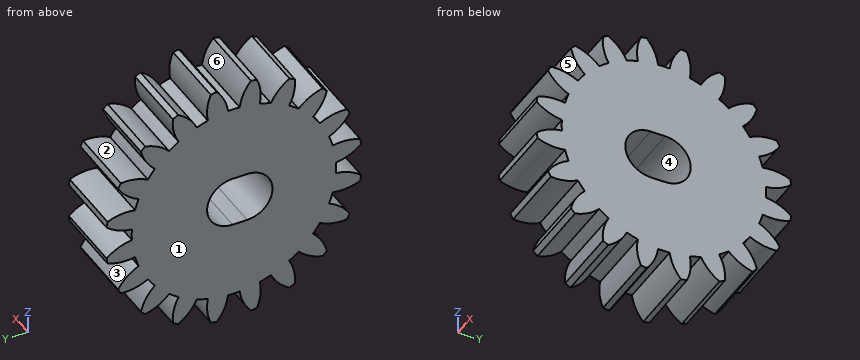
from build123d import *

# Parameters (mm, degrees)
EXTRUDE_1_DEPTH = 6


with BuildPart() as part:
    # Эскиз1 → Бобышка-Вытянуть1 (new body)
    with BuildSketch(Plane(origin=(0.204923016, 3.152126199, 1.20502958), x_dir=(0, 0, -1), z_dir=(1, 0, 0))):
        with BuildLine():
            ThreePointArc((-9.696984117, -1.687169764), (-8.686522764, -2.334065374), (-7.529675738, -2.652202191))
            ThreePointArc((-7.529675738, -2.652202191), (-7.54397042, -3.152126199), (-7.529675738, -3.652050206))
            ThreePointArc((-7.529675738, -3.652050206), (-8.686522764, -3.970187024), (-9.696984117, -4.617082634))
            ThreePointArc((-9.696984117, -4.617082634), (-9.659542166, -4.872905314), (-9.616098021, -5.12777734))
            ThreePointArc((-9.616098021, -5.12777734), (-8.45519043, -5.430761896), (-7.256653844, -5.375842598))
            ThreePointArc((-7.256653844, -5.375842598), (-7.115763881, -5.855715883), (-6.947683816, -6.326754568))
            ThreePointArc((-6.947683816, -6.326754568), (-7.949601035, -6.986806052), (-8.710705152, -7.914290068))
            ThreePointArc((-8.710705152, -7.914290068), (-8.596042186, -8.146021696), (-8.475964561, -8.374994418))
            ThreePointArc((-8.475964561, -8.374994418), (-7.278248455, -8.304409679), (-6.155343422, -7.88181015))
            ThreePointArc((-6.155343422, -7.88181015), (-5.873060104, -8.294659371), (-5.567647504, -8.690704186))
            ThreePointArc((-5.567647504, -8.690704186), (-6.316560278, -9.628059899), (-6.753804986, -10.745343722))
            ThreePointArc((-6.753804986, -10.745343722), (-6.573145013, -10.930300792), (-6.388187943, -11.110960765))
            ThreePointArc((-6.388187943, -11.110960765), (-5.27090412, -10.673716057), (-4.333548407, -9.924803283))
            ThreePointArc((-4.333548407, -9.924803283), (-3.937503592, -10.230215883), (-3.524654371, -10.512499201))
            ThreePointArc((-3.524654371, -10.512499201), (-3.9472539, -11.635404234), (-4.017838639, -12.83312034))
            ThreePointArc((-4.017838639, -12.83312034), (-3.788865917, -12.953197965), (-3.557134289, -13.067860931))
            ThreePointArc((-3.557134289, -13.067860931), (-2.629650273, -12.306756814), (-1.969598789, -11.304839595))
            ThreePointArc((-1.969598789, -11.304839595), (-1.498560104, -11.47291966), (-1.018686819, -11.613809623))
            ThreePointArc((-1.018686819, -11.613809623), (-1.073606117, -12.812346209), (-0.770621561, -13.9732538))
            ThreePointArc((-0.770621561, -13.9732538), (-0.515749535, -14.016697945), (-0.259926855, -14.054139896))
            ThreePointArc((-0.259926855, -14.054139896), (0.386968755, -13.043678543), (0.705105573, -11.886831517))
            ThreePointArc((0.705105573, -11.886831517), (1.20502958, -11.901126199), (1.704953588, -11.886831517))
            ThreePointArc((1.704953588, -11.886831517), (2.023090405, -13.043678543), (2.669986015, -14.054139896))
            ThreePointArc((2.669986015, -14.054139896), (2.925808695, -14.016697945), (3.180680722, -13.9732538))
            ThreePointArc((3.180680722, -13.9732538), (3.483665277, -12.812346209), (3.428745979, -11.613809623))
            ThreePointArc((3.428745979, -11.613809623), (3.908619264, -11.47291966), (4.379657949, -11.304839595))
            ThreePointArc((4.379657949, -11.304839595), (5.039709433, -12.306756814), (5.967193449, -13.067860931))
            ThreePointArc((5.967193449, -13.067860931), (6.198925077, -12.953197965), (6.427897799, -12.83312034))
            ThreePointArc((6.427897799, -12.83312034), (6.35731306, -11.635404234), (5.934713531, -10.512499201))
            ThreePointArc((5.934713531, -10.512499201), (6.347562752, -10.230215883), (6.743607567, -9.924803283))
            ThreePointArc((6.743607567, -9.924803283), (7.68096328, -10.673716057), (8.798247103, -11.110960765))
            ThreePointArc((8.798247103, -11.110960765), (8.983204173, -10.930300792), (9.163864146, -10.745343722))
            ThreePointArc((9.163864146, -10.745343722), (8.726619438, -9.628059899), (7.977706664, -8.690704186))
            ThreePointArc((7.977706664, -8.690704186), (8.283119264, -8.294659371), (8.565402582, -7.88181015))
            ThreePointArc((8.565402582, -7.88181015), (9.688307615, -8.304409679), (10.886023721, -8.374994418))
            ThreePointArc((10.886023721, -8.374994418), (11.006101346, -8.146021696), (11.120764313, -7.914290068))
            ThreePointArc((11.120764313, -7.914290068), (10.359660195, -6.986806052), (9.357742976, -6.326754568))
            ThreePointArc((9.357742976, -6.326754568), (9.525823041, -5.855715883), (9.666713005, -5.375842598))
            ThreePointArc((9.666713005, -5.375842598), (10.86524959, -5.430761896), (12.026157182, -5.12777734))
            ThreePointArc((12.026157182, -5.12777734), (12.069601327, -4.872905314), (12.107043277, -4.617082634))
            ThreePointArc((12.107043277, -4.617082634), (11.096581924, -3.970187024), (9.939734898, -3.652050206))
            ThreePointArc((9.939734898, -3.652050206), (9.95402958, -3.152126199), (9.939734898, -2.652202191))
            ThreePointArc((9.939734898, -2.652202191), (11.096581924, -2.334065374), (12.107043277, -1.687169764))
            ThreePointArc((12.107043277, -1.687169764), (12.069601327, -1.431347083), (12.026157182, -1.176475057))
            ThreePointArc((12.026157182, -1.176475057), (10.86524959, -0.873490502), (9.666713005, -0.9284098))
            ThreePointArc((9.666713005, -0.9284098), (9.525823041, -0.448536515), (9.357742976, 0.02250217))
            ThreePointArc((9.357742976, 0.02250217), (10.359660195, 0.682553654), (11.120764313, 1.61003767))
            ThreePointArc((11.120764313, 1.61003767), (11.006101346, 1.841769298), (10.886023721, 2.07074202))
            ThreePointArc((10.886023721, 2.07074202), (9.688307615, 2.000157281), (8.565402582, 1.577557752))
            ThreePointArc((8.565402582, 1.577557752), (8.283119264, 1.990406973), (7.977706664, 2.386451788))
            ThreePointArc((7.977706664, 2.386451788), (8.726619438, 3.323807501), (9.163864146, 4.441091324))
            ThreePointArc((9.163864146, 4.441091324), (8.983204173, 4.626048394), (8.798247103, 4.806708367))
            ThreePointArc((8.798247103, 4.806708367), (7.68096328, 4.369463659), (6.743607567, 3.620550885))
            ThreePointArc((6.743607567, 3.620550885), (6.347562752, 3.925963485), (5.934713531, 4.208246803))
            ThreePointArc((5.934713531, 4.208246803), (6.35731306, 5.331151836), (6.427897799, 6.528867942))
            ThreePointArc((6.427897799, 6.528867942), (6.198925077, 6.648945567), (5.967193449, 6.763608534))
            ThreePointArc((5.967193449, 6.763608534), (5.039709433, 6.002504416), (4.379657949, 5.000587197))
            ThreePointArc((4.379657949, 5.000587197), (3.908619264, 5.168667262), (3.428745979, 5.309557226))
            ThreePointArc((3.428745979, 5.309557226), (3.483665277, 6.508093811), (3.180680722, 7.669001403))
            ThreePointArc((3.180680722, 7.669001403), (2.925808695, 7.712445548), (2.669986015, 7.749887498))
            ThreePointArc((2.669986015, 7.749887498), (2.023090405, 6.739426145), (1.704953588, 5.582579119))
            ThreePointArc((1.704953588, 5.582579119), (1.20502958, 5.596873801), (0.705105573, 5.582579119))
            ThreePointArc((0.705105573, 5.582579119), (0.386968755, 6.739426145), (-0.259926855, 7.749887498))
            ThreePointArc((-0.259926855, 7.749887498), (-0.515749535, 7.712445548), (-0.770621561, 7.669001403))
            ThreePointArc((-0.770621561, 7.669001403), (-1.073606117, 6.508093811), (-1.018686819, 5.309557226))
            ThreePointArc((-1.018686819, 5.309557226), (-1.498560104, 5.168667262), (-1.969598789, 5.000587197))
            ThreePointArc((-1.969598789, 5.000587197), (-2.629650273, 6.002504416), (-3.557134289, 6.763608534))
            ThreePointArc((-3.557134289, 6.763608534), (-3.788865917, 6.648945567), (-4.017838639, 6.528867942))
            ThreePointArc((-4.017838639, 6.528867942), (-3.9472539, 5.331151836), (-3.524654371, 4.208246803))
            ThreePointArc((-3.524654371, 4.208246803), (-3.937503592, 3.925963485), (-4.333548407, 3.620550885))
            ThreePointArc((-4.333548407, 3.620550885), (-5.27090412, 4.369463659), (-6.388187943, 4.806708367))
            ThreePointArc((-6.388187943, 4.806708367), (-6.573145013, 4.626048394), (-6.753804986, 4.441091324))
            ThreePointArc((-6.753804986, 4.441091324), (-6.316560278, 3.323807501), (-5.567647504, 2.386451788))
            ThreePointArc((-5.567647504, 2.386451788), (-5.873060104, 1.990406973), (-6.155343422, 1.577557752))
            ThreePointArc((-6.155343422, 1.577557752), (-7.278248455, 2.000157281), (-8.475964561, 2.07074202))
            ThreePointArc((-8.475964561, 2.07074202), (-8.596042186, 1.841769298), (-8.710705152, 1.61003767))
            ThreePointArc((-8.710705152, 1.61003767), (-7.949601035, 0.682553654), (-6.947683816, 0.02250217))
            ThreePointArc((-6.947683816, 0.02250217), (-7.115763881, -0.448536515), (-7.256653844, -0.9284098))
            ThreePointArc((-7.256653844, -0.9284098), (-8.45519043, -0.873490502), (-9.616098021, -1.176475057))
            ThreePointArc((-9.616098021, -1.176475057), (-9.659542166, -1.431347083), (-9.696984117, -1.687169764))
        make_face()
        with BuildLine():
            Line((3.38002958, -3.033706418), (3.38002958, -4.283706418))
            ThreePointArc((3.38002958, -4.283706418), (1.20502958, -6.458706418), (-0.96997042, -4.283706418))
            Line((-0.96997042, -4.283706418), (-0.96997042, -3.033706418))
            ThreePointArc((-0.96997042, -3.033706418), (1.20502958, -0.858706418), (3.38002958, -3.033706418))
        make_face(mode=Mode.SUBTRACT)
    extrude(amount=-EXTRUDE_1_DEPTH)


solid = part.part
Verification items for the finished model (mm, model axes). Face numbers are marked on the shaded views. A direction names the side the tool comes from. Coordinates: 2 decimals unless noted, no trailing zeros. Loops run counter-clockwise (first coordinate to the right, second up) from the corner with the lowest first, then second, coordinate; pieces in that order, holes last. Notation, with made-up numbers: (32.25, 42) -> (77.25, 42) arc R22 ccw to (77.25, 77) -> close; hole circle Ø1 at (81, 0.25). An arc over 180 degrees is marked (long way). Write each question's results on one line, items separated by ' | '.
Item 1: Mould release check, pull along Y, two halves, no side actions. Record for the marked faces 1, 2 and 3: +Y half, -Y half, draft (parallel to the pull), parting line (faces both ways), or undercut.
Found:
face 1: draft | face 2: undercut | face 3: +Y half
Item 2: Tool access check on the marked faces 4, 5 and 6. Record the directions out of +Z, -Z, +X, -X, +Y, -Y that give a thin tool (end or side, any length) a straight path to the whole face; none if there is none.
Found:
face 4: +X, -X | face 5: +X, -X, -Y | face 6: +Z, +X, -X
Item 3: Section check A-A, the plane z = 0. Enter the section's corners in (x, y).
Found:
outline: (-5.8, -8.75) -> (0.2, -8.75) -> (0.2, -3.31) -> (-5.8, -3.31) -> close; (-5.8, 2.29) -> (0.2, 2.29) -> (0.2, 8.75) -> (-5.8, 8.75) -> close
Item 4: Gauge pin test, flat ends, axial feed: pin 1 (3 mm diameter, centred on x = -1.5, z = -2, fed in from -Y); pin 2 (1.5 mm diameter, centred on x = -4.5, z = 3.5, fed in from -Y); pin 3 (1.4 mm diameter, centred on x = -2.5, y = -0.5, fed in from +Z); pin 4 (2 mm diameter, centred on x = -2, y = 3.5, fed in from +Z). Record the tip position at first contact, or that the pin passes through.
Found:
pin 1: stops at y = -10.9 | pin 2: stops at y = -9.55 | pin 3: stops at z = 10.57 | pin 4: stops at z = 9.75
Item 5: Section check B-B, the plane y = -6.5. Enter the section's corners in (x, z), plus the area to 3 significant figures.
Found:
outline: (-5.8, -7.54) -> (0.2, -7.54) -> (0.2, 7.54) -> (-5.8, 7.54) -> close | area: 90.4 mm2
Item 6: Material ranges on L1, parallel to Y at x = -0.5, z = 7.25; L2, parallel to Z at x = -4.05, y = -3.5, recorded low to high.
Found:
L1: y = -7.86 to -6.07, -4.9 to 4.9, 6.07 to 7.86 | L2: z = -8.73 to 8.73
Item 7: Section check C-C, the plane z = -2.75. Enter the section's corners in (x, y), plus the area to 3 significant figures.
Found:
outline: (-5.8, -8.31) -> (0.2, -8.31) -> (0.2, 8.31) -> (-5.8, 8.31) -> close | area: 99.7 mm2
